from build123d import *

# Parameters (mm, degrees)
EXTRUDE_1_DEPTH      = 8.5
EXTRUDE_1_DEPTH_BACK = 8.5
SKETCH_3_R           = 2
CUT_EXTRUDE_2_DEPTH  = 15.5
SKETCH_4_R           = 2
CUT_EXTRUDE_3_DEPTH  = 15.5
FILLET_1_R           = 8.5
CHAMFER_1_SIZE       = 1.5


with BuildPart() as part:
    # 草图1 → 凸台-拉伸1 (new, two sides: drawn at the far end of the back side and taken through both)
    with BuildSketch(Plane(origin=(0, 0, 0), x_dir=(0, 0, -1), z_dir=(1, 0, 0)).offset(-EXTRUDE_1_DEPTH_BACK)):
        with BuildLine():
            Line((-40, 0), (-3, 0))
            ThreePointArc((-3, 0), (-0.878679656, 0.878679656), (0, 3))
            Line((0, 3), (0, 40))
            Line((0, 40), (-2, 40))
            Line((-2, 40), (-2, 3))
            ThreePointArc((-2, 3), (-2.292893219, 2.292893219), (-3, 2))
            Line((-3, 2), (-40, 2))
            Line((-40, 2), (-40, 0))
        make_face()
    extrude(amount=EXTRUDE_1_DEPTH + EXTRUDE_1_DEPTH_BACK)

    # 草图3 → 切除-拉伸2 (cut)
    with BuildSketch(Plane(origin=(0, 2, 0), x_dir=(1, 0, 0), z_dir=(0, 1, 0))):
        with Locations(Location((0, -33, 0), (0, 0, 270))):
            Circle(SKETCH_3_R)
        with Locations(Location((0, -16, 0), (0, 0, 270))):
            Circle(SKETCH_3_R)
    extrude(amount=-CUT_EXTRUDE_2_DEPTH, mode=Mode.SUBTRACT)

    # 草图4 → 切除-拉伸3 (cut)
    with BuildSketch(Plane.XY.offset(2)):
        with Locations((0, 33)):
            Circle(SKETCH_4_R)
        with Locations((0, 16)):
            Circle(SKETCH_4_R)
    extrude(amount=-CUT_EXTRUDE_3_DEPTH, mode=Mode.SUBTRACT)

    # 圆角1
    fillet_1_edges = [part.edges().sort_by_distance(p)[0] for p in [
        (8.5, 40, 1),
        (-8.5, 40, 1),
        (8.5, 1, 40),
        (-8.5, 1, 40),
    ]]
    fillet(fillet_1_edges, radius=FILLET_1_R - 0.0001)  # a hair under: the kernel refuses the full size

    # 倒角1
    chamfer_1_edges = [part.edges().sort_by_distance(p)[0] for p in [
        (0, 2, 31),
        (0, 2, 14),
        (-2, 33, 2),
        (-2, 16, 2),
    ]]
    chamfer(chamfer_1_edges, length=CHAMFER_1_SIZE)


solid = part.part
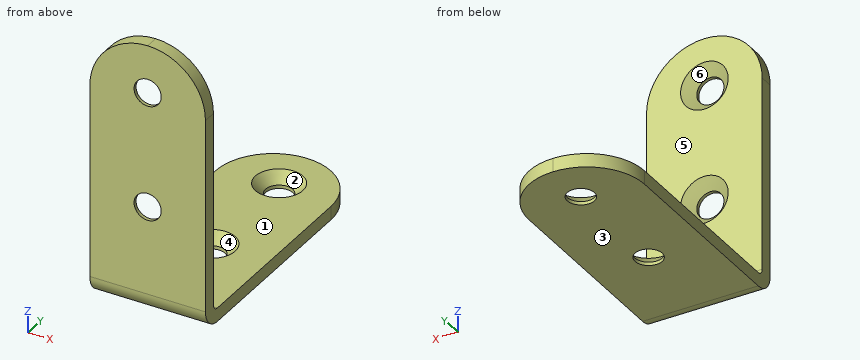
Can you work these out from the model? Positions are in its coordinate system, mm. Face numbers are marked on the shaded views. A direction names the side the tool comes from. Round coordinates to 2 decimals unless told otherwise and drop trailing zeros. Loops run counter-clockwise (first coordinate to the right, second up) from the corner with the lowest first, then second, coordinate; pieces in that order, holes last. Notation, with made-up numbers: (21.25, -15.5) - (62.25, -15.5) arc R18 cw to (62.25, 7.5) - close; hole circle Ø10 at (-12.75, -32.75). An arc over 180 degrees is marked (long way). Answer in a Markdown table with one row per item. Add a question column.
Q1. I want a section at A-A on z = 16. List the corners of the cut face in (x, y) for me.
Q2. Which directions (+Z, -Z, +X, -X, +Y, -Y) give clear straight access to the entire face, cutting with the end or side of a thin tool? Please do the marked faces 1 and 2.
Q3. I want a section at C-C on y = 3.5. List the corners of the cut face in (x, z) for me, and give its area (3 significant figures).
Q4. I need wall thicknesses on L1, parallel to Y at x = 0, z = 0.45; L2, parallel to Y at x = -2, z = 19. Which ranges of each line are inside material? Lowest first, please.
Q5. I want a section at D-D on x = -6.75. List the corners of the cut face in (y, z) for me, and give its area (3 significant figures).
Q6. We'd pull the mould along Z, two halves only. Please class the marked faces 3, 4, 5 and 6: pulls with the +Z half, pulls with the -Z half, needs draft (parallel to the pull), parting line crosses it, or undercut.
Q7. For pin 1 Ø6.5 at (x, z) = (0, 33) entering from +Y; pin 2 Ø4.5 at (x, y) = (0, 16) entering from +Z; pin 3 Ø1.5 at (x, y) = (-3, 35.5) entering from +Z, each with a flat end and sliding along its axis, tell me the tip position at first contact or that it passes through.
A:
| question | item | result |
|---|---|---|
| 1 | outline | (-8.5, 0) - (-2, 0) - (-2, 0.5) - (-3.5, 2) - (-8.5, 2) - close; (2, 0) - (8.5, 0) - (8.5, 2) - (3.5, 2) - (2, 0.5) - close |
| 2 | face 1 | +Z, +X, -X, +Y |
| 2 | face 2 | +Z |
| 3 | outline | (-8.5, 0) - (8.5, 0) - (8.5, 2) - (-8.5, 2) - close |
| 3 | area | 34.0 mm^2 |
| 4 | L1 | 1.42 to 14, 18 to 31, 35 to 40 |
| 4 | L2 | 0 to 2 |
| 5 | outline | (0, 3) arc R3 ccw to (3, 0) - (36.67, 0) - (36.67, 2) - (3, 2) arc R1 cw to (2, 3) - (2, 36.67) - (0, 36.67) - close |
| 5 | area | 141 mm^2 |
| 6 | face 3 | pulls with the -Z half |
| 6 | face 4 | pulls with the +Z half |
| 6 | face 5 | needs draft |
| 6 | face 6 | undercut |
| 7 | pin 1 | y = 1.75 |
| 7 | pin 2 | z = 0.75 |
| 7 | pin 3 | z = 2 |
